Autodesk Fusion 360 part; units mm, degrees
sketch "Sketch1" plane through (0, 0, 0) normal (0, 1, 0) x (1, 0, 0)
  line L0 (-18.1, 70) -> (20, 70)
  line L1 (20, 70) -> (20, -57)
  line L2 (20, -57) -> (-18.1, -57)
  line L3 (-18.1, -57) -> (-18.1, 70)
  dimension "d1" = 127
  dimension "d2" = 38.1
extrude "Extrude1" add sketch "Sketch1" along normal blind 25.4
sketch "Sketch2" plane through (0, 25.4, 0) normal (0, 1, 0) x (-1, 0, 0)
  line L0 (18.1, 57) -> (-20, 57)
  line L1 (-20, 57) -> (-20, -70)
  line L2 (-20, -70) -> (18.1, -70)
  line L3 (18.1, -70) -> (18.1, 57)
  line L4 (18.1, 57) -> (-20, 57)
  line L5 (-20, 57) -> (-20, 25.25)
  line L6 (-20, 25.25) -> (18.1, 25.25)
  line L7 (18.1, 25.25) -> (18.1, 57)
  line L8 (18.1, -70) -> (-20, -70)
  line L9 (-20, -70) -> (-20, -38.25)
  line L10 (-20, -38.25) -> (18.1, -38.25)
  line L11 (18.1, -38.25) -> (18.1, -70)
  dimension "d5" = 31.75
  dimension "d6" = 31.75
extrude "Extrude2" cut sketch "Sketch2" against normal blind 12.7 contours L0 L1 L3 L4 L5 L6 L7 | L1 L2 L3 L8 L9 L10 L11
sketch "Sketch3" plane through (0, 12.7, 0) normal (0, 1, 0) x (-1, 0, 0)
  line L0 (18.1, 25.25) -> (18.1, 57)
  line L1 (18.1, 57) -> (-20, 57)
  line L2 (-20, 57) -> (-20, 25.25)
  line L3 (-20, 25.25) -> (18.1, 25.25)
  circle A0 centre (8.575, 41.125) radius 3.175
  circle A1 centre (-10.475, 41.125) radius 3.175
  dimension "d9" = 6.35
  dimension "d10" = 15.875
  dimension "d12" = 6.35
  dimension "d13" = 15.875
  dimension "d15" = 19.05
  dimension "d16" = 9.525
extrude "Extrude3" cut sketch "Sketch3" against normal blind 30 contours A0 | A1
sketch "Sketch4" plane through (0, 12.7, 0) normal (0, 1, 0) x (-1, 0, 0)
  line L0 (18.1, -38.25) -> (-20, -38.25)
  line L1 (-20, -38.25) -> (-20, -70)
  line L2 (-20, -70) -> (18.1, -70)
  line L3 (18.1, -70) -> (18.1, -38.25)
sketch "Sketch5" plane through (0, 12.7, 0) normal (0, 1, 0) x (-1, 0, 0)
  circle A0 centre (-10.475, -54.125) radius 3.175
  circle A1 centre (8.575, -54.125) radius 3.175
  line L0 (-20, -38.25) -> (-20, -70)
  line L1 (-20, -70) -> (18.1, -70)
  dimension "d19" = 6.35
  dimension "d20" = 6.35
  dimension "d21" = 9.525
  dimension "d22" = 19.05
  dimension "d23" = 15.875
  dimension "d24" = 15.875
extrude "Extrude4" cut sketch "Sketch5" against normal blind 40
sketch "Sketch6" plane through (0, 25.4, 0) normal (0, 1, 0) x (-1, 0, 0)
  line L0 (18.1, 25.25) -> (-20, 25.25)
  line L1 (-20, 25.25) -> (-20, -38.25)
  line L2 (-20, -38.25) -> (18.1, -38.25)
  line L3 (18.1, -38.25) -> (18.1, 25.25)
  line L4 (9.55, -20) -> (-11.45, -20)
  line L5 (-11.45, -20) -> (-11.45, 7)
  line L6 (-11.45, 7) -> (9.55, 7)
  line L7 (9.55, 7) -> (9.55, -20)
  circle A0 centre (-0.95, 16.125) radius 6.35
  circle A1 centre (-0.95, -29.125) radius 6.35
  dimension "d27" = 21
  dimension "d28" = 27
  dimension "d29" = 18.25
  dimension "d30" = 8.55
  dimension "d31" = 12.7
  dimension "d32" = 9.125
  dimension "d33" = 19.05
  dimension "d34" = 12.7
  dimension "d35" = 9.125
  dimension "d36" = 19.05
extrude "Extrude5" cut sketch "Sketch6" against normal blind 4 contours L4 L5 L6 L7 | A0 | A1
sketch "Sketch7" plane through (0, 25.4, 0) normal (0, 1, 0) x (-1, 0, 0)
  line L0 (-11.45, -20) -> (-11.45, 7)
  line L1 (-11.45, 7) -> (9.55, 7)
  line L2 (9.55, 7) -> (9.55, -20)
  line L3 (9.55, -20) -> (-11.45, -20)
  circle A0 centre (-0.95, 16.125) radius 6.35
  circle A1 centre (-0.95, -29.125) radius 6.35
  line L4 (18.1, 25.25) -> (-20, 25.25)
  line L5 (-20, 25.25) -> (-20, -38.25)
  line L6 (-20, -38.25) -> (18.1, -38.25)
  line L7 (18.1, -38.25) -> (18.1, 25.25)
  circle A2 centre (-0.95, -29.125) radius 6.35
  circle A3 centre (-0.95, 16.125) radius 6.35
  dimension "d39" = 12.7
  dimension "d40" = 12.7
extrude "Extrude6" cut sketch "Sketch7" against normal blind 12.7 contours A0 A3 | A1 A2
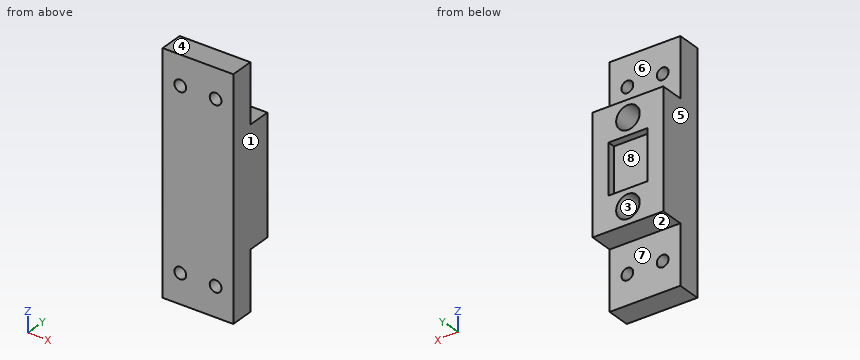
Geometry check sheet. Reference: the model listing, model coordinates, mm. Face numbers are marked on the shaded views. A direction names the side the tool comes from. Coordinates: 2 decimals unless noted, no trailing zeros. Order: outer loops, then holes, each group sorted by start corner. A loop starts at its lowest first (then second) coordinate and runs counter-clockwise, first axis right, second up. Notation, with made-up numbers: M 2,46 L 16,46 A25 cw 16,81 Z; hole C 61.5,81 d4. An arc over 180 degrees is marked long. One line per question, with ' | ' between items. Start each with the question number.
Item 1: Cross-section at A-A on x = 15. Enter the section's corners in (y, z), then the cut area to 3 significant figures.
Item 2: Gauge pin test, flat ends, axial feed: pin 1 (6.5 mm diameter, centred on x = 8.5, y = 19, fed in from +Z); pin 2 (8 mm diameter, centred on y = 18, z = 33, fed in from -X); pin 3 (3 mm diameter, centred on x = 6, y = 24, fed in from -Z); pin 4 (7.5 mm diameter, centred on x = 0.95, z = 16.125, fed in from +Y). Record the tip position at first contact, or that the pin passes through.
Item 3: Cross-section at B-B on x = 10. Enter the section's corners in (y, z), then the cut area to 3 significant figures.
Item 4: Set-up check for the marked faces 5, 6, 7 and 8: record each of +Z, -Z, +X, -X, +Y, -Y from which the full face is reachable in a straight line by a thin tool's end or side.
Item 5: Material ranges on L1, parallel to Z at x = 0.95, y = 19 (3 decimals); L2, parallel to X at y = 24, z = 1; L3, parallel to X at y = 8.75, z = 43, recorded low to high. Write a range as [from, to].
Item 6: Draft check along Z on the marked faces 1, 2, 3 and 4. Enter one of: pulls with the +Z half, pulls with the -Z half, needs draft (parallel to the pull), parting line crosses it, or undercut.
Item 7: Cross-section at C-C on y = 8.25. Enter the section's corners in (x, z) (3 decimals).
Item 8: Cross-section at D-D on z = 28.5. Enter the section's corners in (x, y), then the cut area to 3 significant figures.
Findings:
1) outline: M 0,-70 L 12.7,-70 L 12.7,-38.25 L 25.4,-38.25 L 25.4,25.25 L 12.7,25.25 L 12.7,57 L 0,57 Z | area: 2,420 mm²
2) pin 1: stops at z = 25.25 | pin 2: passes through | pin 3: stops at z = -38.25 | pin 4: stops at y = 12.7
3) outline: M 0,-70 L 12.7,-70 L 12.7,-57.26 L 0,-57.26 Z; M 0,-50.99 L 12.7,-50.99 L 12.7,-38.25 L 25.4,-38.25 L 25.4,-20 L 21.4,-20 L 21.4,7 L 25.4,7 L 25.4,25.25 L 12.7,25.25 L 12.7,37.99 L 0,37.99 Z; M 0,44.26 L 12.7,44.26 L 12.7,57 L 0,57 Z | area: 2,150 mm²
4) face 5: +Z, -Z, -X, +Y, -Y | face 6: +Z, +X, -X, +Y | face 7: -Z, +X, -X, +Y | face 8: +Y
5) L1: z = [-38.25, -35.475], [-22.775, 9.775], [22.475, 25.25] | L2: x = [-18.1, -9.55], [11.45, 20] | L3: x = [-18.1, -11.14], [-6.01, 7.91], [13.04, 20]
6) face 1: needs draft | face 2: pulls with the -Z half | face 3: undercut | face 4: pulls with the +Z half
7) outline: M -18.1,-70 L 20,-70 L 20,57 L -18.1,57 Z; hole C -8.575,-54.125 d6.35; hole C -8.575,41.125 d6.35; hole C 10.475,-54.125 d6.35; hole C 10.475,41.125 d6.35
8) outline: M -18.1,0 L 20,0 L 20,12.7 L -18.1,12.7 Z | area: 484 mm²
